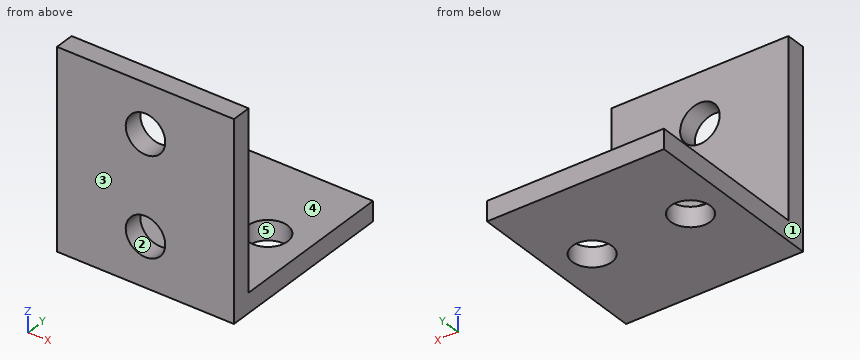
from build123d import *

# Parameters (mm, degrees)
SKETCH1_W           = 22.86
SKETCH1_H           = 25.4
BOSS_EXTRUDE1_DEPTH = 24.13
SKETCH2_W           = 22.86
SKETCH2_H           = 21.59
CUT_EXTRUDE1_DEPTH  = 42.832959494
SKETCH3_R           = 2.5527
CUT_EXTRUDE2_DEPTH  = 41.421129376
SKETCH4_R           = 2.5527
CUT_EXTRUDE3_DEPTH  = 41.341245643


with BuildPart() as part:
    # Sketch1 → Boss-Extrude1 (new body)
    with BuildSketch(Plane(origin=(0, 0, 0), x_dir=(1, 0, 0), z_dir=(0, 1, 0))):
        with Locations((11.43, 12.7)):
            Rectangle(SKETCH1_W, SKETCH1_H)
    extrude(amount=BOSS_EXTRUDE1_DEPTH)

    # Sketch2 → Cut-Extrude1 (cut, through all)
    with BuildSketch(Plane(origin=(22.86, 0, 0), x_dir=(0, 0, -1), z_dir=(1, 0, 0))):
        with Locations((11.43, 13.335)):
            Rectangle(SKETCH2_W, SKETCH2_H)
    extrude(amount=-CUT_EXTRUDE1_DEPTH, mode=Mode.SUBTRACT)

    # Sketch3 → Cut-Extrude2 (cut, through all)
    with BuildSketch(Plane(origin=(0, 2.54, 0), x_dir=(1, 0, 0), z_dir=(0, 1, 0))):
        with Locations(Location((11.43, 6.35, 0), (0, 0, 270))):
            Circle(SKETCH3_R)
        with Locations(Location((11.43, 19.05, 0), (0, 0, 270))):
            Circle(SKETCH3_R)
    extrude(amount=-CUT_EXTRUDE2_DEPTH, mode=Mode.SUBTRACT)

    # Sketch4 → Cut-Extrude3 (cut, through all)
    with BuildSketch(Plane.XY.offset(-22.86)):
        with Locations((17.78, 12.7)):
            Circle(SKETCH4_R)
        with Locations((5.08, 12.7)):
            Circle(SKETCH4_R)
    extrude(amount=-CUT_EXTRUDE3_DEPTH, mode=Mode.SUBTRACT)


solid = part.part
The listing builds one solid part. Answer for the finished solid, in the listing's coordinates (mm). Face numbers are marked on the shaded views. A direction names the side the tool comes from. Give positions to 0.01 mm unless a question says otherwise; leave off trailing zeros. Order: outer loops, then holes, each group sorted by start corner. A loop starts at its lowest first (then second) coordinate and runs counter-clockwise, first axis right, second up. Notation, with made-up numbers: (71.5, 23.25) -> (125.5, 23.25) arc R16 ccw to (125.5, 38.25) -> close; hole circle Ø5 at (33.5, 38.5). An arc over 180 degrees is marked (long way). Put each result on its own line as item: value.
Item 1: For the marked faces 4 and 5, determine the directions among +Z, -Z, +X, -X, +Y, -Y from which every point of the face is accessible in a straight line to the end or side of a thin tool.
Established:
face 4: +Z, +X, -X, +Y
face 5: +Z, -Z
Item 2: For a pull along X with two mould halves and no side action, classify the marked faces 1, 2 and 3 as released by +X, released by -X, zero draft, split by the parting line, or undercut.
Established:
face 1: released by -X
face 2: undercut
face 3: zero draft
Item 3: A cutting plane is placed at B-B on z = -19.05. Give the vertices of the cut face in (x, y), plus the area to 3 significant figures.
Established:
outline: (0, 0) -> (8.88, 0) -> (8.88, 2.54) -> (0, 2.54) -> close; (13.98, 0) -> (22.86, 0) -> (22.86, 2.54) -> (13.98, 2.54) -> close
area: 45.1 mm^2
Item 4: A cutting plane is placed at C-C on y = 12.7. Give the vertices of the cut face in (x, z).
Established:
outline: (0, -25.4) -> (2.53, -25.4) -> (2.53, -22.86) -> (0, -22.86) -> close; (7.63, -25.4) -> (15.23, -25.4) -> (15.23, -22.86) -> (7.63, -22.86) -> close; (20.33, -25.4) -> (22.86, -25.4) -> (22.86, -22.86) -> (20.33, -22.86) -> close
Item 5: A cutting plane is placed at D-D on x = 11.43. Give the vertices of the cut face in (y, z).
Established:
outline: (0, -25.4) -> (24.13, -25.4) -> (24.13, -22.86) -> (2.54, -22.86) -> (2.54, -21.6) -> (0, -21.6) -> close; (0, -16.5) -> (2.54, -16.5) -> (2.54, -8.9) -> (0, -8.9) -> close; (0, -3.8) -> (2.54, -3.8) -> (2.54, 0) -> (0, 0) -> close
Item 6: A cutting plane is placed at A-A on x = 5.08. Give the vertices of the cut face in (y, z), plus the area to 3 significant figures.
Established:
outline: (0, -25.4) -> (10.15, -25.4) -> (10.15, -22.86) -> (2.54, -22.86) -> (2.54, 0) -> (0, 0) -> close; (15.25, -25.4) -> (24.13, -25.4) -> (24.13, -22.86) -> (15.25, -22.86) -> close
area: 106 mm^2
Item 7: Given P1, Ø11, axis at x = 13, y = 10, coming from the +Z side; P2, Ø8, axis at y = 13.5, z = -16, coming from the +X side; P3, Ø5, axis at x = 4.5, z = -4.5, coming from the +Y side, each flat-ended and moving along its own axis, determine where each tip first touches the part or whether it passes through.
Established:
P1: stops at z = -22.86
P2: passes through
P3: stops at y = 2.54
Item 8: Straight lines are drawn through the part: line 1 (X direction, y = 0.9, z = -19.05); line 2 (Z direction, x = 13.75, y = 13.75); line 3 (Y direction, x = 1, z = -15.5). For each, find the intervals that lie inside material, in ascending order.
Established:
line 1: x = 0 to 8.88, 13.98 to 22.86
line 2: z = -25.4 to -22.86
line 3: y = 0 to 2.54
